from build123d import *

# Parameters (mm, degrees)
F0_R     = 10
F1_DEPTH = 50
F2_SIZE  = 2
F4_DEPTH = 50


with BuildPart() as f1:
    # F0 (on Front) → F1 (new body)
    with BuildSketch(Plane.XZ):
        Circle(F0_R)
    extrude(amount=-F1_DEPTH)

    # F2
    f2_edges = [f1.edges().sort_by_distance(p)[0] for p in [
        (-10, 50, 0),
        (-10, 0, 0),
    ]]
    chamfer(f2_edges, length=F2_SIZE)

    # F3 (on face) → F4 (cut, through all)
    with BuildSketch(Plane(origin=(0, 50, 0), x_dir=(-1, 0, 0), z_dir=(0, 1, 0))):
        with BuildLine():
            Line((-1, 5), (-1, 3.872983))
            ThreePointArc((-1, 3.872983), (0, -4), (1, 3.872983))
            Line((1, 3.872983), (1, 5))
            Line((1, 5), (-1, 5))
        make_face()
    extrude(amount=-F4_DEPTH, mode=Mode.SUBTRACT)


solid = f1.part
Verification items for the finished model (mm, model axes). A direction names the side the tool comes from. Give positions to 0.01 mm unless a question says otherwise; leave off trailing zeros. Write each loop counter-clockwise with the first axis right and the second up, starting at its lowest first coordinate (ties: lowest second). Pieces come first, ordered by that corner, then holes. Notation, with made-up numbers: M 33.5,26.5 L 43.5,26.5 A32 cw 43.5,63.5 Z; hole C -7,-27.75 d2. An arc over 180 degrees is marked long. Put each result on its own line as item: value. Start each with the question number.
1. Scan lines: line 1 along Z through (x, y) = (0, 30.5); line 2 along X through (y, z) = (8, 4); line 3 along X through (y, z) = (34, -1). Record each from-to range of solid material in increasing order. Write a range as [from, to].
2. Section check A-A (x = 0). Record the cut outline in (y, z), and give its area (3 significant figures).
3. Set-up check for faces 1 (the face through (-4, 50, -2)), 2 (the face through (1, 25.4, 4.4)): record each of +Z, -Z, +X, -X, +Y, -Y from which the full face is reachable in a straight line by a thin tool's end or side.
4. Section check C-C (y = 25.5). Record the cut outline in (x, z), and give its area (3 significant figures).
5. Section check B-B (z = 0). Record the cut outline in (x, y).
6. Go/stop test with flat-tipped pins: pin 1 Ø0.6 at (y, z) = (22, 4.5) entering from +X; pin 2 Ø1 at (x, y) = (-4, 18.5) entering from -Z; pin 3 Ø5 at (x, y) = (-6.5, 30) entering from +Z; pin 4 Ø6.5 at (x, z) = (0, 0) entering from +Y. Record where each tip stops, or that it passes through.
7. Draft check along Z on faces 3 (the face through (-1, 25.4, 4.4)), 4 (the face through (-2.17, 24.68, -9.76)), 5 (the face through (-4, 0, -2)). Enter one of: +Z half, -Z half, draft (parallel to the pull), parting line (faces both ways), or undercut.
Answer list:
1. line 1: [-10, -4], [5, 10]
1. line 2: [-9.17, -1], [1, 9.17]
1. line 3: [-9.95, -3.87], [3.87, 9.95]
2. outline: M 0,-8 L 2,-10 L 48,-10 L 50,-8 L 50,-4 L 0,-4 Z; M 0,5 L 50,5 L 50,8 L 48,10 L 2,10 L 0,8 Z
2. area: 542 mm2
3. face 1: +Z, -Z, +X, -X, +Y
3. face 2: +Y, -Y
4. outline: C 0,0 d20; hole M -1,3.87 A4 ccw long 1,3.87 L 1,5 L -1,5 Z
4. area: 262 mm2
5. outline: M -10,2 L -8,0 L -4,0 L -4,50 L -8,50 L -10,48 Z; M 4,0 L 8,0 L 10,2 L 10,48 L 8,50 L 4,50 Z
6. pin 1: x = 9.08
6. pin 2: z = -9.37
6. pin 3: z = 9.17
6. pin 4: through
7. face 3: undercut
7. face 4: parting line
7. face 5: draft
